from build123d import *

# Parameters (mm, degrees)
ESBO_O1_W                = 62
ESBO_O1_H                = 102
RESSALTO_EXTRUS_O1_DEPTH = 48
FILETE1_R                = 4
CASCA1_T                 = -2
ESBO_O2_R                = 12.5
CORTE_EXTRUS_O1_DEPTH    = 94.536089292
ESBO_O3_R                = 12.5
CORTE_EXTRUS_O2_DEPTH    = 117.914498673
ESBO_O4_R                = 1.25
RESSALTO_EXTRUS_O2_DEPTH = 10


with BuildPart() as part:
    # Esboço1 → Ressalto-extrusão1 (new body)
    with BuildSketch(Plane.XY):
        Rectangle(ESBO_O1_W, ESBO_O1_H)
    extrude(amount=RESSALTO_EXTRUS_O1_DEPTH)

    # Filete1
    filete1_edges = [part.edges().sort_by_distance(p)[0] for p in [
        (0, -51, 0),
        (-31, 0, 0),
        (0, 51, 0),
        (31, 0, 0),
        (31, -51, 24),
        (-31, -51, 24),
        (-31, 51, 24),
        (31, 51, 24),
    ]]
    fillet(filete1_edges, radius=FILETE1_R)

    # Casca1
    casca1_openings = [part.faces().sort_by_distance(p)[0] for p in [
        (0, 0, 48),
    ]]
    offset(amount=CASCA1_T, openings=casca1_openings, kind=Kind.INTERSECTION)

    # Esboço2 → Corte-extrusão1 (cut, through all)
    with BuildSketch(Plane.ZY.offset(31)):
        with Locations((20, 0)):
            Circle(ESBO_O2_R)
        with Locations((20, 30)):
            Circle(ESBO_O2_R)
        with Locations((20, -30)):
            Circle(ESBO_O2_R)
    extrude(amount=-CORTE_EXTRUS_O1_DEPTH, mode=Mode.SUBTRACT)

    # Esboço3 → Corte-extrusão2 (cut, through all)
    with BuildSketch(Plane(origin=(0, 51, 0), x_dir=(1, 0, 0), z_dir=(0, 1, 0))):
        with Locations(Location((0, -20, 0), (0, 0, 270))):
            Circle(ESBO_O3_R)
    extrude(amount=-CORTE_EXTRUS_O2_DEPTH, mode=Mode.SUBTRACT)

    # Esboço4 → Ressalto-extrusão2 (add)
    # profile 1 of 2: a face of its own
    with BuildSketch(Plane.XY.offset(48)):
        with BuildLine():
            Line((-4.5, 42), (-4.5, 49))
            Line((-4.5, 49), (4.5, 49))
            Line((4.5, 49), (4.5, 42))
            ThreePointArc((4.5, 42), (0, 37.5), (-4.5, 42))
        make_face()
        with Locations((0, 42)):
            Circle(ESBO_O4_R, mode=Mode.SUBTRACT)
    # profile 2 of 2: a face of its own
    with BuildSketch(Plane.XY.offset(48)):
        with BuildLine():
            Line((4.5, -49), (-4.5, -49))
            Line((-4.5, -49), (-4.5, -42))
            ThreePointArc((-4.5, -42), (0, -37.5), (4.5, -42))
            Line((4.5, -42), (4.5, -49))
        make_face()
        with Locations(Location((0, -42, 0), (0, 0, 180))):
            Circle(ESBO_O4_R, mode=Mode.SUBTRACT)
    extrude(amount=-RESSALTO_EXTRUS_O2_DEPTH)


solid = part.part
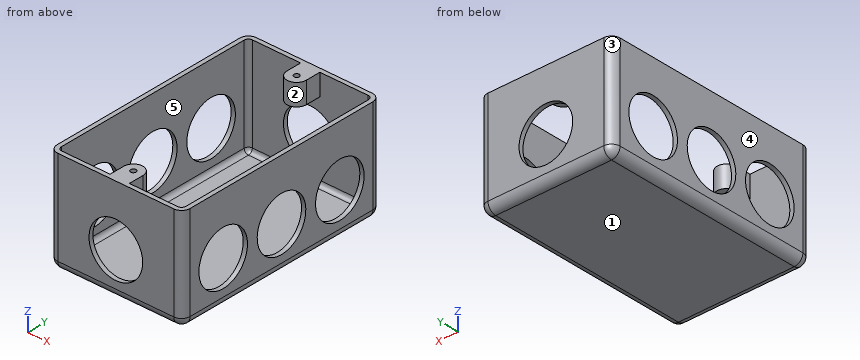
Check sheet for the modelled part. Datum: model origin and axes. Units: mm. Face numbers are marked on the shaded views. A direction names the side the tool comes from. Give positions to 0.01 mm unless a question says otherwise; leave off trailing zeros. Loops run counter-clockwise (first coordinate to the right, second up) from the corner with the lowest first, then second, coordinate; pieces in that order, holes last. Notation, with made-up numbers: M 3.5,-39.5 L 17.5,-39.5 A29 cw 17.5,-11.5 Z; hole C -33.5,44.25 d7. An arc over 180 degrees is marked long. Use a Markdown table: item, result. Add a question column.
Q1. Sectioned sample at B-B, the plane z = 36.5. Record the cut outline in (x, y).
Q2. Sectioned sample at D-D, the plane y = 15. Record the cut outline in (x, z).
Q3. Go/stop test with flat-tipped pins: pin 1 (6 mm diameter, centred on x = 24.5, y = 7.5, fed in from +Z); pin 2 (22.5 mm diameter, centred on x = 0, z = 20, fed in from +Y); pin 3 (1 mm diameter, centred on x = 6, y = -19, fed in from +Z). Record where each tip stops, or that it passes through.
Q4. Mould release check, pull along X, two halves, no side actions. Record for the marked faces 1, 2 and 3: pulls with the +X half, pulls with the -X half, needs draft (parallel to the pull), parting line crosses it, or undercut.
Q5. Sectioned sample at A-A, the plane y = -30. Record the cut outline in (x, z), then the cut area to 3 significant figures.
Q6. Tool access check on the marked faces 4 and 5. Record the directions out of +Z, -Z, +X, -X, +Y, -Y that give a thin tool (end or side, any length) a straight path to the whole face; none if there is none.
Q7. Sectioned sample at C-C, the plane x = 0. Give the number of separate pieces and of enclosed holes in the cut face, then the cut area to 3 significant figures.
Q8. Scan lines: line 1 along X through (y, z) = (-42, 42); line 2 along X through (y, z) = (-24, 42); line 3 along Y through (x, z) = (-23, 16.5). Record each from-to range of solid material in increasing order. Write a range as [from, to].
Verdict:
| question | item | result |
|---|---|---|
| 1 | outline | M -31,-47 A4 ccw -27,-51 L 27,-51 A4 ccw 31,-47 L 31,47 A4 ccw 27,51 L -27,51 A4 ccw -31,47 Z; hole M -29,-47 A2 ccw -27,-49 L 27,-49 A2 ccw 29,-47 L 29,47 A2 ccw 27,49 L -27,49 A2 ccw -29,47 Z |
| 2 | outline | M -31,4 A4 ccw -27,0 L 27,0 A4 ccw 31,4 L 31,48 L 29,48 L 29,4 A2 cw 27,2 L -27,2 A2 cw -29,4 L -29,48 L -31,48 Z |
| 3 | pin 1 | z = 2.06 |
| 3 | pin 2 | through |
| 3 | pin 3 | z = 2 |
| 4 | face 1 | needs draft |
| 4 | face 2 | undercut |
| 4 | face 3 | pulls with the -X half |
| 5 | outline | M -31,4 A4 ccw -27,0 L 27,0 A4 ccw 31,4 L 31,7.5 L 29,7.5 L 29,4 A2 cw 27,2 L -27,2 A2 cw -29,4 L -29,7.5 L -31,7.5 Z; M -31,32.5 L -29,32.5 L -29,48 L -31,48 Z; M 29,32.5 L 31,32.5 L 31,48 L 29,48 Z |
| 5 | area | 203 mm^2 |
| 6 | face 4 | +Z, -Z, -X, +Y, -Y |
| 6 | face 5 | +Z |
| 7 | separate pieces | 5 |
| 7 | enclosed holes | 0 |
| 7 | area | 463 mm^2 |
| 8 | line 1 | [-31, -29], [-4.5, -1.25], [1.25, 4.5], [29, 31] |
| 8 | line 2 | [-31, -29], [29, 31] |
| 8 | line 3 | [-51, -49], [49, 51] |
